Model file for the job. Use its own axes, mm. Face numbers are marked on the shaded views. A direction names the side the tool comes from. Give positions to 0.01 mm unless a question says otherwise; leave off trailing zeros. Write each loop counter-clockwise with the first axis right and the second up, starting at its lowest first coordinate (ties: lowest second). Pieces come first, ordered by that corner, then holes. Notation, with made-up numbers: M -10,56 L 5,56 A34 ccw 5,86 Z; hole C 85,-22.5 d3. An arc over 180 degrees is marked long. Answer as a JSON object with one key per item and string values. Group by question number.
```python
from build123d import *

# Parameters (mm, degrees)
SKETCH1_R               = 33.655
SKETCH1_R_2             = 28.575
BOSS_EXTRUDE1_DEPTH     = 12.7
SKETCH2_R               = 39.37
BOSS_EXTRUDE2_DEPTH     = 5.08
SKETCH3_R               = 5.08
CUT_EXTRUDE1_DEPTH      = 1
CUT_EXTRUDE1_DEPTH_BACK = 18.78


with BuildPart() as part:
    # Sketch1 → Boss-Extrude1 (new body)
    with BuildSketch(Plane(origin=(0, 0, 0), x_dir=(1, 0, 0), z_dir=(0, 1, 0))):
        Circle(SKETCH1_R)
        Circle(SKETCH1_R_2, mode=Mode.SUBTRACT)
    extrude(amount=BOSS_EXTRUDE1_DEPTH)

    # Sketch2 → Boss-Extrude2 (add)
    with BuildSketch(Plane(origin=(0, 12.7, 0), x_dir=(1, 0, 0), z_dir=(0, 1, 0))):
        Circle(SKETCH2_R)
    extrude(amount=BOSS_EXTRUDE2_DEPTH)

    # Sketch3 → Cut-Extrude1 (cut, two sides)
    with BuildSketch(Plane(origin=(0, 17.78, 0), x_dir=(1, 0, 0), z_dir=(0, 1, 0))) as cut_extrude1_sk:
        Circle(SKETCH3_R)
    extrude(amount=CUT_EXTRUDE1_DEPTH, mode=Mode.SUBTRACT)
    extrude(cut_extrude1_sk.sketch, amount=-CUT_EXTRUDE1_DEPTH_BACK, mode=Mode.SUBTRACT)


solid = part.part
```
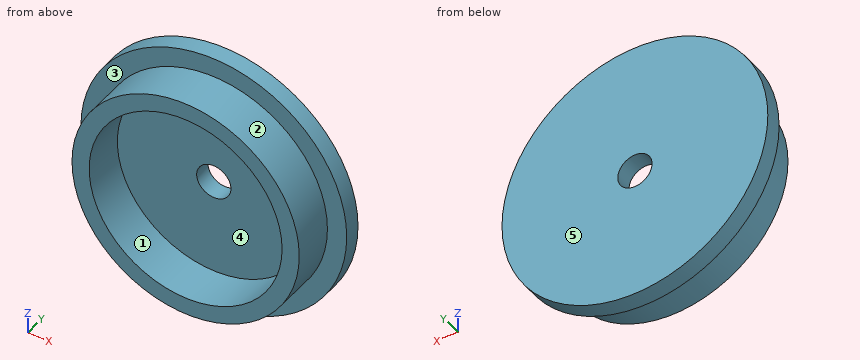
Q1. Slice it at B-B, the plane z = 0. Write the cut outline in (x, y) (3 decimals).
Q2. Wall check: L1, parallel to X at y = 3.5, z = 0 (3 decimals); L2, parallel to X at y = 15.2, z = 0. Give the ranges that are in metal, low to high.
Q3. Two-plate mould, pull along Z, no slides. Class the marked faces 1, 2 and 3: +Z half, -Z half, draft (parallel to the pull), parting line (faces both ways), or undercut.
Q4. Slice it at A-A, the plane x = 0. Write the cut outline in (y, z) (3 decimals).
Q5. Drop flat-ended pins along their axis: P1, Ø2, axis at x = 25, y = 2, coming from the +Z side; P2, Ø6, axis at y = 10, z = -17.5, coming from the -X side; P3, Ø4, axis at y = 8.5, z = 1, coming from the +X side (3 decimals); P4, Ø9, axis at x = 0, z = 0, coming from the -Y side. Give the stop position or say it passes through.
Q6. Slice it at D-D, the plane z = 12. Write the cut outline in (x, y).
Q7. 3-axis set-ups, long thin cutter, end or side, ignore diameter. For the marked faces 4 and 5: which of +Z, -Z, +X, -X, +Y, -Y reach the whole face in a straight line?
Q8. Slice it at C-C, the plane y = 15. Write the cut outline in (x, z).
Solved:
{
 "1": {"outline": "M -39.37,12.7 L -33.655,12.7 L -33.655,0 L -28.575,0 L -28.575,12.7 L -5.08,12.7 L -5.08,17.78 L -39.37,17.78 Z; M 5.08,12.7 L 28.575,12.7 L 28.575,0 L 33.655,0 L 33.655,12.7 L 39.37,12.7 L 39.37,17.78 L 5.08,17.78 Z"},
 "2": {"L1": "x = -33.655 to -28.575, 28.575 to 33.655", "L2": "x = -39.37 to -5.08, 5.08 to 39.37"},
 "3": {"face 1": "undercut", "face 2": "parting line", "face 3": "draft"},
 "4": {"outline": "M 0,-33.655 L 12.7,-33.655 L 12.7,-39.37 L 17.78,-39.37 L 17.78,-5.08 L 12.7,-5.08 L 12.7,-28.575 L 0,-28.575 Z; M 0,28.575 L 12.7,28.575 L 12.7,5.08 L 17.78,5.08 L 17.78,39.37 L 12.7,39.37 L 12.7,33.655 L 0,33.655 Z"},
 "5": {"P1": "stops at z = 23.59", "P2": "stops at x = -35.89", "P3": "stops at x = 33.655", "P4": "passes through"},
 "6": {"outline": "M -37.5,12.7 L -31.44,12.7 L -31.44,0 L -25.93,0 L -25.93,12.7 L 25.93,12.7 L 25.93,0 L 31.44,0 L 31.44,12.7 L 37.5,12.7 L 37.5,17.78 L -37.5,17.78 Z"},
 "7": {"face 4": "-Y", "face 5": "+Z, -Z, +X, -X, +Y"},
 "8": {"outline": "C 0,0 d78.74; hole C 0,0 d10.16"}
}
